```python
from build123d import *

# Parameters (mm, degrees)
SKIZZE1_W                       = 271
SKIZZE1_H                       = 70
AUFSATZ_LINEAR_AUSTRAGEN1_DEPTH = 5
SKIZZE2_W                       = 72
SKIZZE2_H                       = 70
SCHNITT_LINEAR_AUSTRAGEN1_DEPTH = 3
SKIZZE3_R                       = 4
SCHNITT_LINEAR_AUSTRAGEN2_DEPTH = 10
SKIZZE4_R                       = 2.5
SCHNITT_LINEAR_AUSTRAGEN3_DEPTH = 10
SKIZZE5_R                       = 2.5
SCHNITT_LINEAR_AUSTRAGEN4_DEPTH = 10
SKIZZE6_R                       = 2
SCHNITT_LINEAR_AUSTRAGEN5_DEPTH = 10
SKIZZE7_R                       = 4
SCHNITT_LINEAR_AUSTRAGEN6_DEPTH = 10
SKIZZE8_R                       = 2
SCHNITT_LINEAR_AUSTRAGEN7_DEPTH = 10


with BuildPart() as part:
    # Skizze1 → Aufsatz-Linear austragen1 (new body)
    with BuildSketch(Plane.XY):
        with Locations((135.5, 35)):
            Rectangle(SKIZZE1_W, SKIZZE1_H)
    extrude(amount=AUFSATZ_LINEAR_AUSTRAGEN1_DEPTH)

    # Skizze2 → Schnitt-Linear austragen1 (cut)
    with BuildSketch(Plane.XY.offset(5)):
        with Locations((78.5, 35)):
            Rectangle(SKIZZE2_W, SKIZZE2_H)
    extrude(amount=-SCHNITT_LINEAR_AUSTRAGEN1_DEPTH, mode=Mode.SUBTRACT)

    # Skizze3 → Schnitt-Linear austragen2 (cut)
    with BuildSketch(Plane(origin=(0, 0, 0), x_dir=(-1, 0, 0), z_dir=(0, 0, -1))):
        with Locations((-48.5, 37)):
            Circle(SKIZZE3_R)
        with Locations((-108.5, 37)):
            Circle(SKIZZE3_R)
        with Locations((-108.5, 7)):
            Circle(SKIZZE3_R)
        with Locations((-48.5, 7)):
            Circle(SKIZZE3_R)
    extrude(amount=-SCHNITT_LINEAR_AUSTRAGEN2_DEPTH, mode=Mode.SUBTRACT)

    # Skizze4 → Schnitt-Linear austragen3 (cut)
    with BuildSketch(Plane(origin=(0, 0, 0), x_dir=(-1, 0, 0), z_dir=(0, 0, -1))):
        with Locations((-234.5, 23.5)):
            Circle(SKIZZE4_R)
        with Locations((-266.5, 23.5)):
            Circle(SKIZZE4_R)
    extrude(amount=-SCHNITT_LINEAR_AUSTRAGEN3_DEPTH, mode=Mode.SUBTRACT)

    # Skizze5 → Schnitt-Linear austragen4 (cut)
    with BuildSketch(Plane(origin=(0, 0, 0), x_dir=(-1, 0, 0), z_dir=(0, 0, -1))):
        with Locations((-36.5, 23.5)):
            Circle(SKIZZE5_R)
        with Locations((-4.5, 23.5)):
            Circle(SKIZZE5_R)
    extrude(amount=-SCHNITT_LINEAR_AUSTRAGEN4_DEPTH, mode=Mode.SUBTRACT)

    # Skizze6 → Schnitt-Linear austragen5 (cut)
    with BuildSketch(Plane(origin=(0, 0, 0), x_dir=(-1, 0, 0), z_dir=(0, 0, -1))):
        with Locations((-10, 60)):
            Circle(SKIZZE6_R)
        with Locations((-50, 60)):
            Circle(SKIZZE6_R)
        with Locations((-161, 60)):
            Circle(SKIZZE6_R)
        with Locations((-221, 60)):
            Circle(SKIZZE6_R)
        with Locations((-261, 60)):
            Circle(SKIZZE6_R)
        with Locations((-107, 60)):
            Circle(SKIZZE6_R)
    extrude(amount=-SCHNITT_LINEAR_AUSTRAGEN5_DEPTH, mode=Mode.SUBTRACT)

    # Skizze7 → Schnitt-Linear austragen6 (cut)
    with BuildSketch(Plane(origin=(0, 0, 0), x_dir=(-1, 0, 0), z_dir=(0, 0, -1))):
        with Locations((-211.5, 40)):
            Circle(SKIZZE7_R)
    extrude(amount=-SCHNITT_LINEAR_AUSTRAGEN6_DEPTH, mode=Mode.SUBTRACT)

    # Skizze8 → Schnitt-Linear austragen7 (cut)
    with BuildSketch(Plane(origin=(0, 0, 0), x_dir=(-1, 0, 0), z_dir=(0, 0, -1))):
        with Locations((-150, 60)):
            Circle(SKIZZE8_R)
    extrude(amount=-SCHNITT_LINEAR_AUSTRAGEN7_DEPTH, mode=Mode.SUBTRACT)


solid = part.part
```
Input: part model. Units: mm. Frame: model coordinates. A direction names the side the tool comes from. Give positions to 0.01 mm unless a question says otherwise; leave off trailing zeros. Order: outer loops, then holes, each group sorted by start corner. A loop starts at its lowest first (then second) coordinate and runs counter-clockwise, first axis right, second up. Notation, with made-up numbers: (14.5, 27) - (61.5, 27) arc R15 cw to (61.5, 52) - close; hole circle Ø9 at (17, -1.5). An arc over 180 degrees is marked (long way). One line per item, written item: value.
1. Cut plane A-A, the plane y = 23.5. Output: boundary loops of the cut face in (x, z), and give its area (3 significant figures).
Determined:
outline: (0, 0) - (2, 0) - (2, 5) - (0, 5) - close; (7, 0) - (34, 0) - (34, 5) - (7, 5) - close; (39, 0) - (232, 0) - (232, 5) - (114.5, 5) - (114.5, 2) - (42.5, 2) - (42.5, 5) - (39, 5) - close; (237, 0) - (264, 0) - (264, 5) - (237, 5) - close; (269, 0) - (271, 0) - (271, 5) - (269, 5) - close
area: 1,040 mm2
2. Pin query (flat end, axial travel): pin 1 Ø3 at (x, y) = (4.5, 23.5) entering from +Z; pin 2 Ø9 at (x, y) = (48.5, 7) entering from +Z. Return the tip coordinate at first contact, or that it passes through.
Determined:
pin 1: through
pin 2: z = 2
3. Cut plane D-D, the plane x = 102. Output: boundary loops of the cut face in (y, z), and give its area (3 significant figures).
Determined:
outline: (0, 0) - (70, 0) - (70, 2) - (0, 2) - close
area: 140 mm2
4. Cut plane B-B, the plane z = 4.25. Give the number of separate pieces and of enclosed holes in the cut face, and give its area (3 significant figures).
Determined:
separate pieces: 2
enclosed holes: 10
area: 13,700 mm2
5. Draft query along Y for faces 1 (the face through (112.496, 7.176, 0.986)), 2 (the face through (21, 35, 5)), 3 (the face through (134, 70, 2)). Return one class per face: released by +Y, released by -Y, zero draft, split by the parting line, or undercut.
Determined:
face 1: undercut
face 2: zero draft
face 3: released by +Y
6. Reachability of faces 4 (the face through (134, 0, 2)), 5 (the face through (78, 35, 2)) from +Z, -Z, +X, -X, +Y, -Y: full face, straight path, thin tool, end or side. Return the list, or none.
Determined:
face 4: +Z, -Z, +X, -X, -Y
face 5: +Z, +Y, -Y
7. Line query: probe 1 along Y at (x, z) = (221, 1.6); probe 2 along X at (y, z) = (29.5, 4.55); probe 3 along Y at (x, z) = (107, 0.45). Output: solid intervals per line, ascending.
Determined:
probe 1: 0 to 58, 62 to 70
probe 2: 0 to 42.5, 114.5 to 271
probe 3: 0 to 3.29, 10.71 to 33.29, 40.71 to 58, 62 to 70
8. Cut plane C-C, the plane y = 64.5. Output: boundary loops of the cut face in (x, z), and give its area (3 significant figures).
Determined:
outline: (0, 0) - (271, 0) - (271, 5) - (114.5, 5) - (114.5, 2) - (42.5, 2) - (42.5, 5) - (0, 5) - close
area: 1,140 mm2
